Part model, mm, in its own coordinate system. Face numbers are marked on the shaded views. A direction names the side the tool comes from. Round coordinates to 2 decimals unless told otherwise and drop trailing zeros. Order: outer loops, then holes, each group sorted by start corner. A loop starts at its lowest first (then second) coordinate and runs counter-clockwise, first axis right, second up. Notation, with made-up numbers: M 46.5,2 L 97.5,2 A16 ccw 97.5,26 Z; hole C 22.25,84.25 d8. An arc over 180 degrees is marked long. One line per question, with ' | ' between items.
from build123d import *

# Parameters (mm, degrees)
F1_DEPTH    = 10
F2_R        = 2.65
F2_R_2      = 2.7
F3_DEPTH    = 10.001
F4_T1_DEPTH = 74
F6_DEPTH    = 7


# Not quite as in the source:
# - a fillet or chamfer that OpenCascade refuses, or shapes differently, is made with other operations: its cross-section is extruded or revolved along the edge and cut away or added


with BuildPart() as f1:
    # F0 (on Top) → F1 (new body)
    with BuildSketch(Plane.XY):
        with BuildLine():
            Line((-33.8368600405, -9.2521366523), (-50.8368600405, -9.1521366523))
            Line((-50.8368600405, -9.1521366523), (-50.8368600405, -21.2521366523))
            Line((-50.8368600405, -21.2521366523), (1.1631399595, -50.2521366523))
            Line((1.1631399595, -50.2521366523), (1.1631399595, -36.2521366523))
            Line((1.1631399595, -36.2521366523), (0.8274590919, -30.2521366523))
            ThreePointArc((0.8274590919, -30.2521366523), (-4.1287803642, -19.2185823544), (-13.8368600405, -12.003541191))
            Line((-13.8368600405, -12.003541191), (-21.8368600405, -10.1521366523))
            ThreePointArc((-21.8368600405, -10.1521366523), (-27.8233098501, -9.521467447), (-33.8368600405, -9.2521366523))
        make_face()
    extrude(amount=F1_DEPTH)

    # F2 (on face) → F3 (cut, through all)
    with BuildSketch(Plane.XY.offset(10)):
        with Locations((-43.8368600405, -17.1521366523)):
            Circle(F2_R)
        with Locations((-16.8368600405, -20.2521366523)):
            Circle(F2_R)
        with Locations((-4.8368600405, -41.2521366523)):
            Circle(F2_R)
        with Locations((-10.8368600405, -29.2521366523)):
            Circle(F2_R_2)
    extrude(amount=-F3_DEPTH, mode=Mode.SUBTRACT)

    # F4: fillet of radius 5 on 1 edges, made by hand

    # F4_s2 → F4_t1 (cut)
    with BuildSketch(Plane.XZ.offset(6.2521366523)):
        with BuildLine():
            ThreePointArc((-3.8368600405, 0), (-0.3013261345, 1.4644660941), (1.1631399595, 5))
            Line((1.1631399595, 5), (1.2631399595, 5))
            Line((1.2631399595, 5), (1.2631399595, -0.1))
            Line((1.2631399595, -0.1), (-3.8368600405, -0.1))
            Line((-3.8368600405, -0.1), (-3.8368600405, 0))
        make_face()
    extrude(amount=F4_T1_DEPTH, mode=Mode.SUBTRACT)

    # F5 (on face) → F6 (cut)
    with BuildSketch(Plane.XY.offset(10)):
        Polygon((-28.5395178944, -11.904838495), (-48.1065809727, -11.4794680849), (-48.1065809727, -19.3488299847), (-9.8231984302, -41.8934859335), (-2.166522434, -32.4289835989), (-5.6758336723, -22.3264265805), (-14.7149646655, -14.1380364075), align=None)
    extrude(amount=-F6_DEPTH, mode=Mode.SUBTRACT)


solid = f1.part
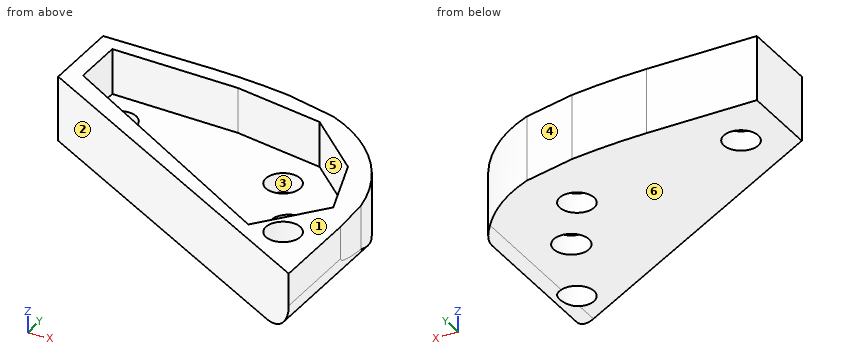
1) Saw through at D-D (x = -37). List the corners of the cut face in (y, z), plus the area to 3 significant figures.
The answers:
outline: M -28.97,0 L -9.23,0 L -9.23,10 L -11.72,10 L -11.72,3 L -25.89,3 L -25.89,10 L -28.97,10 Z | area: 98.2 mm²
2) Drop flat-ended pins along their axis: pin 1 (1 mm diameter, centred on y = -46, z = 9, fed in from -X); pin 2 (8 mm diameter, centred on x = -12.5, y = -23, fed in from +Z); pin 3 (8.5 mm diameter, centred on x = -43.84, y = -17.15, fed in from +Z); pin 4 (2 mm diameter, centred on x = -4.5, z = 6, fed in from +Y). Give the stop position or say it passes through.
The answers:
pin 1: stops at x = -7.36 | pin 2: stops at z = 3 | pin 3: stops at z = 10 | pin 4: stops at y = -17.66
3) Which spindle directions (+Z, -Z, +X, -X, +Y, -Y) get a long thin tool onto all of the face, cutting with end or side? Do the marked faces 5 and 6. Say none if no direction does.
The answers:
face 5: +Z | face 6: -Z, +X, -X, +Y, -Y
4) Saw through at A-A (x = -3). List the corners of the cut face in (y, z).
The answers:
outline: M -47.93,0.07 L -43.16,0.07 L -43.16,10 L -47.93,10 Z; M -39.34,0.07 L -20.74,0.07 L -20.74,10 L -30.03,10 L -30.03,3 L -33.46,3 L -33.46,10 L -39.34,10 Z
5) Saw through at B-B (y = -28). List the corners of the cut face in (x, z), plus the area to 3 significant figures.
The answers:
outline: M -38.74,0 L -13.23,0 L -13.23,3 L -33.42,3 L -33.42,10 L -38.74,10 Z; M -8.44,0 L -3.84,0 A5 ccw 0.33,2.24 L 0.33,10 L -3.71,10 L -3.71,3 L -8.44,3 Z | area: 166 mm²
6) Saw through at C-C (z = 8.75). List the corners of the cut face in (x, y), plus the area to 3 significant figures.
The answers:
outline: M -50.84,-21.25 L 1.16,-50.25 L 1.16,-36.25 L 0.83,-30.25 A24 ccw -13.84,-12 L -21.84,-10.15 A100 ccw -33.84,-9.25 L -50.84,-9.15 Z; hole M -48.11,-19.35 L -9.82,-41.89 L -2.17,-32.43 L -5.68,-22.33 L -14.71,-14.14 L -28.54,-11.9 L -48.11,-11.48 Z; hole C -4.84,-41.25 d5.3 | area: 417 mm²
7) Probe line 1 (Z direction, x = -18.5, y = -27); line 2 (X direction, y = -42, z = 6.25); line 3 (Y direction, x = -5.5, z = 1.5). List the from-to ranges inside material, lowest first. Write a range as [from, to].
The answers:
line 1: z = [0, 3] | line 2: x = [-13.63, -7.38], [-2.29, 1.16] | line 3: y = [-46.54, -43.82], [-38.69, -17.66]
8) Two-plate mould, pull along Y, no slides. Class the marked faces 1, 2, 3 and 4: released by +Y, released by -Y, zero draft, split by the parting line, or undercut.
The answers:
face 1: zero draft | face 2: released by -Y | face 3: undercut | face 4: released by +Y
